Read the model definition and answer for the solid it produces. Units are mm, in the model's axes. A direction names the side the tool comes from. Coordinates: 2 decimals unless noted, no trailing zeros. Write each loop counter-clockwise with the first axis right and the second up, starting at its lowest first coordinate (ties: lowest second). Pieces come first, ordered by that corner, then holes. Notation, with made-up numbers: (-28.5, 88) -> (4.5, 88) arc R23 cw to (4.5, 100) -> close; hole circle Ø10 at (68.5, -8.5). An arc over 180 degrees is marked (long way). Answer in a Markdown table with one row per item. Add a question column.
Item 1: Which of the six approach directions +Z, -Z, +X, -X, +Y, -Y give full straight-line access (tool end or side, diameter ignored) to faces 5 (the face through (61, 0, 15)), 6 (the face through (-58.6, -47.1, 47.1)), 7 (the face through (60, -47, 53)), 8 (the face through (-63, 0, 9)), 9 (the face through (3, 37, 2))?
Item 2: Section B-B on y = 42.5 is taken. Write down the section's boundary in (x, z).
Item 3: For a pull along Z with two mould halves and no side action, classify faces 1 (the face through (-1, -1, 0)), 2 (the face through (-62, 34, 20)), 3 (the face through (-60, -1, 11)), 4 (the face through (-61, 39, 40)) as +Z half, -Z half, draft (parallel to the pull), parting line (faces both ways), or undercut.
Item 4: Section A-A on z = 38 is taken. Write down the section's boundary in (x, y), then the cut area to 3 significant figures.
Item 5: Given pin 1 Ø2.5 at (x, y) = (62, 0.5) entering from +Z; pin 2 Ø6 at (y, z) = (-21, 18.5) entering from -X; pin 3 Ø4 at (x, y) = (21, -34.5) entering from +Z, each flat-ended and moving along its own axis, determine where each tip first touches the part or whether it passes through.
Item 6: Section D-D on z = 23 is taken. Write down the section's boundary in (x, y), then the cut area to 3 significant figures.
Item 7: Section C-C on x = 40.5 is taken. Write down the section's boundary in (y, z).
Item 8: Straight lines are drawn through the part: line 1 (Z direction, x = 0, y = -57.1); line 2 (X direction, y = -56, z = 48); line 3 (X direction, y = 42, z = 25). For each, find the intervals that lie inside material, in ascending order. Write a range as from..to.
```python
from build123d import *

# Parameters (mm, degrees)
SKETCH1_W           = 126
SKETCH1_H           = 110
BOSS_EXTRUDE1_DEPTH = 3
SKETCH2_W           = 50
SKETCH2_H           = 16
BOSS_EXTRUDE2_DEPTH = 3
BOSS_EXTRUDE3_DEPTH = 16
BOSS_EXTRUDE4_DEPTH = 16
SKETCH5_W           = 126
SKETCH5_H           = 53
BOSS_EXTRUDE5_DEPTH = 3
SKETCH7_W           = 3
SKETCH7_H           = 78
BOSS_EXTRUDE6_DEPTH = 12
SKETCH8_R           = 2.15
CUT_EXTRUDE1_DEPTH  = 140.810586151
CUT_EXTRUDE2_DEPTH  = 140.810586151
CUT_EXTRUDE3_DEPTH  = 138.397234324
SKETCH11_W          = 3
SKETCH11_H          = 16
BOSS_EXTRUDE7_DEPTH = 2.5
CHAMFER1_SIZE       = 10
CHAMFER2_SIZE       = 2
SKETCH12_W          = 4
SKETCH12_H          = 8
CUT_EXTRUDE4_DEPTH  = 101.445258723
FILLET1_R           = 1
CHAMFER3_SIZE       = 2


with BuildPart() as part:
    # Sketch1 → Boss-Extrude1 (new body)
    with BuildSketch(Plane.XY):
        Rectangle(SKETCH1_W, SKETCH1_H)
    extrude(amount=BOSS_EXTRUDE1_DEPTH)

    # Sketch2 → Boss-Extrude2 (add)
    with BuildSketch(Plane.ZY.offset(63)):
        with Locations((28, 47)):
            Rectangle(SKETCH2_W, SKETCH2_H)
        with Locations((28, -47)):
            Rectangle(SKETCH2_W, SKETCH2_H)
    boss_extrude2 = extrude(amount=-BOSS_EXTRUDE2_DEPTH)

    # Sketch3 → Boss-Extrude3 (add)
    with BuildSketch(Plane.XZ.offset(55)):
        Polygon((-60, 45.5), (-57, 48.5), (-60, 51.5), align=None)
    boss_extrude3 = extrude(amount=-BOSS_EXTRUDE3_DEPTH)

    # Sketch4 → Boss-Extrude4 (add)
    with BuildSketch(Plane(origin=(0, 55, 0), x_dir=(1, 0, 0), z_dir=(0, 1, 0))):
        Polygon((-60, -51.5), (-57, -48.5), (-60, -45.5), align=None)
    boss_extrude4 = extrude(amount=-BOSS_EXTRUDE4_DEPTH)

    # Mirror1: Boss-Extrude2, Boss-Extrude3, Boss-Extrude4 across plane
    add(boss_extrude2.mirror(Plane(origin=(0, 0, 0), x_dir=(0, 0, 1), z_dir=(1, 0, 0))))
    add(boss_extrude3.mirror(Plane(origin=(0, 0, 0), x_dir=(0, 0, 1), z_dir=(1, 0, 0))))
    add(boss_extrude4.mirror(Plane(origin=(0, 0, 0), x_dir=(0, 0, 1), z_dir=(1, 0, 0))))

    # Sketch5 → Boss-Extrude5 (add)
    with BuildSketch(Plane.XZ.offset(55)):
        with Locations((0, 26.5)):
            Rectangle(SKETCH5_W, SKETCH5_H)
    extrude(amount=BOSS_EXTRUDE5_DEPTH)

    # Sketch7 → Boss-Extrude6 (add)
    with BuildSketch(Plane.XY.offset(3)):
        with Locations((-61.5, 0)):
            Rectangle(SKETCH7_W, SKETCH7_H)
        with Locations((61.5, 0)):
            Rectangle(SKETCH7_W, SKETCH7_H)
    extrude(amount=BOSS_EXTRUDE6_DEPTH)

    # Sketch8 → Cut-Extrude1 (cut, through all)
    with BuildSketch(Plane.XZ.offset(58)):
        with Locations(Location((0, 48, 0), (0, 0, 270))):
            Circle(SKETCH8_R)
    extrude(amount=-CUT_EXTRUDE1_DEPTH, mode=Mode.SUBTRACT)

    # Sketch9 → Cut-Extrude2 (cut, through all)
    with BuildSketch(Plane.XZ.offset(58)):
        Polygon((-1.075, 49.861954618), (0, 50.482606158), (1.075, 49.861954618), align=None)
    extrude(amount=-CUT_EXTRUDE2_DEPTH, mode=Mode.SUBTRACT)

    # Sketch10 → Cut-Extrude3 (cut, through all)
    with BuildSketch(Plane(origin=(0, -55, 0), x_dir=(1, 0, 0), z_dir=(0, 1, 0))):
        Polygon((-60, -45.5), (-60, -45.7), (-57.2, -48.5), (-60, -51.3), (-60, -51.5), (-57, -48.5), align=None)
        Polygon((60, -45.7), (57.2, -48.5), (60, -51.3), (60, -51.5), (57, -48.5), (60, -45.5), align=None)
    extrude(amount=CUT_EXTRUDE3_DEPTH, mode=Mode.SUBTRACT)

    # Sketch11 → Boss-Extrude7 (add)
    with BuildSketch(Plane.XY.offset(53)):
        Polygon((-63, -39), (-63, -58), (63, -58), (63, -39), (60, -39), (60, -55), (-60, -55), (-60, -39), align=None)
        with Locations((-61.5, 47)):
            Rectangle(SKETCH11_W, SKETCH11_H)
        with Locations((61.5, 47)):
            Rectangle(SKETCH11_W, SKETCH11_H)
    extrude(amount=BOSS_EXTRUDE7_DEPTH)

    # Chamfer1
    chamfer1_edges = [part.edges().sort_by_distance(p)[0] for p in [
        (-61.5, -39, 15),
        (-61.5, 39, 15),
        (61.5, 39, 15),
        (61.5, -39, 15),
    ]]
    chamfer(chamfer1_edges, length=CHAMFER1_SIZE)

    # Chamfer2
    chamfer2_edges = [part.edges().sort_by_distance(p)[0] for p in [
        (-60, 0, 3),
        (0, -55, 3),
        (60, 0, 3),
    ]]
    chamfer(chamfer2_edges, length=CHAMFER2_SIZE)

    # Sketch12 → Cut-Extrude4 (cut, through all)
    with BuildSketch(Plane.XY.offset(3)):
        with Locations((-5, 37)):
            Rectangle(SKETCH12_W, SKETCH12_H)
        with Locations((5, 37)):
            Rectangle(SKETCH12_W, SKETCH12_H)
    extrude(amount=-CUT_EXTRUDE4_DEPTH, mode=Mode.SUBTRACT)

    # Fillet1
    fillet1_edges = [part.edges().sort_by_distance(p)[0] for p in [
        (-7, 33, 1.5),
        (-7, 41, 1.5),
        (-3, 41, 1.5),
        (-3, 33, 1.5),
        (3, 33, 1.5),
        (3, 41, 1.5),
        (7, 41, 1.5),
        (7, 33, 1.5),
    ]]
    fillet(fillet1_edges, radius=FILLET1_R)

    # Chamfer3
    chamfer3_edges = [part.edges().sort_by_distance(p)[0] for p in [
        (-63, -58, 27.75),
        (63, -58, 27.75),
    ]]
    chamfer(chamfer3_edges, length=CHAMFER3_SIZE)


solid = part.part
```
Results below:
| question | item | result |
|---|---|---|
| 1 | face 5 | +Z, +X, -X |
| 1 | face 6 | +Y |
| 1 | face 7 | +Z, +Y |
| 1 | face 8 | +Z, -Z, -X, +Y, -Y |
| 1 | face 9 | +Z, -Z |
| 2 | outline | (-63, 0) -> (63, 0) -> (63, 55.5) -> (60, 55.5) -> (60, 51.3) -> (57.2, 48.5) -> (60, 45.7) -> (60, 5) -> (58, 3) -> (-58, 3) -> (-60, 5) -> (-60, 45.7) -> (-57.2, 48.5) -> (-60, 51.3) -> (-60, 55.5) -> (-63, 55.5) -> close |
| 3 | face 1 | -Z half |
| 3 | face 2 | +Z half |
| 3 | face 3 | undercut |
| 3 | face 4 | draft |
| 4 | outline | (-63, -56) -> (-61, -58) -> (61, -58) -> (63, -56) -> (63, -39) -> (60, -39) -> (60, -55) -> (-60, -55) -> (-60, -39) -> (-63, -39) -> close; (-63, 39) -> (-60, 39) -> (-60, 55) -> (-63, 55) -> close; (60, 39) -> (63, 39) -> (63, 55) -> (60, 55) -> close |
| 4 | area | 566 mm2 |
| 5 | pin 1 | stops at z = 15 |
| 5 | pin 2 | passes through |
| 5 | pin 3 | stops at z = 3 |
| 6 | outline | (-63, -56) -> (-61, -58) -> (61, -58) -> (63, -56) -> (63, -37) -> (60, -37) -> (60, -55) -> (-60, -55) -> (-60, -37) -> (-63, -37) -> close; (-63, 37) -> (-60, 37) -> (-60, 55) -> (-63, 55) -> close; (60, 37) -> (63, 37) -> (63, 55) -> (60, 55) -> close |
| 6 | area | 590 mm2 |
| 7 | outline | (-58, 0) -> (55, 0) -> (55, 3) -> (-53, 3) -> (-55, 5) -> (-55, 55.5) -> (-58, 55.5) -> close |
| 8 | line 1 | z = 0..45.85, 50.48..55.5 |
| 8 | line 2 | x = -63..-2.15, 2.15..63 |
| 8 | line 3 | x = -63..-60, 60..63 |
